Model file for the job. Use its own axes, mm. Face numbers are marked on the shaded views. A direction names the side the tool comes from. Give positions to 0.01 mm unless a question says otherwise; leave off trailing zeros. Order: outer loops, then holes, each group sorted by start corner. A loop starts at its lowest first (then second) coordinate and runs counter-clockwise, first axis right, second up. Notation, with made-up numbers: (42.5, -36) -> (61.5, -36) arc R35 cw to (61.5, 3) -> close; hole circle Ø6 at (-29, 72). An arc over 180 degrees is marked (long way). Use CSV: the item, a comma, the result in double quotes. Start each with the question number.
1. Cut at C-C on y = 3.5. List the corners of the cut face in (x, z).
2. Wall check: line 1 (X direction, y = 7.5, z = -1.6); line 2 (X direction, y = 6, z = -1.6); line 3 (Z direction, x = -1.5, y = 7.5). Give the ranges that are in metal, low to high. Write a range as from..to.
3. 3-axis set-ups, long thin cutter, end or side, ignore diameter. For the marked faces 5, 6 and 7: which of +Z, -Z, +X, -X, +Y, -Y reach the whole face in a straight line?
4. Cut at B-B on y = 7.5. List the corners of the cut face in (x, z), then the cut area to 3 significant figures.
5. Cut at A-A on y = 1.5. List the corners of the cut face in (x, z), then the cut area to 3 significant figures.
6. Pull direction X, two halves, no side cores. Call the marked faces 1, 2, 3 and 4: released by +X, released by -X, zero draft, split by the parting line, or undercut.
7. Drop flat-ended pins along their axis: pin 1 (3 mm diameter, centred on x = 2.5, z = -4, fed in from -Y); pin 2 (1.9 mm diameter, centred on x = 0, y = 1, fed in from +Z); pin 3 (1.2 mm diameter, centred on x = 0, y = 1, fed in from -Z). Give the stop position or say it passes through.
```python
from build123d import *

# Parameters (mm, degrees)
F3_DEPTH = 3
F4_R     = 2


with BuildPart() as f1:
    # F0 (on Right) → F1 (revolve)
    with BuildSketch(Plane.YZ):
        Polygon((0, 0.6), (0, 0), (3, 0), (3, 2.4), (10, 2.4), (10, 8.4), (0, 8.6), (0, 9), (-1, 9), (-1, 7.61980002), (9, 7.41980002), (9, 3.4), (0.4, 3.4), (0.4, 0.6), align=None)
    revolve(axis=Axis((0, 5.8202521418, -1.6), (0, 1, 0)))

    # F2 (on face) → F3 (join, through all)
    with BuildSketch(Plane(origin=(0, 3, 0), x_dir=(-1, 0, 0), z_dir=(0, 1, 0))):
        with BuildLine():
            Line((-1.1618950039, -0.5), (1.1618950039, -0.5))
            ThreePointArc((1.1618950039, -0.5), (0, 0), (-1.1618950039, -0.5))
        make_face()
        with BuildLine():
            ThreePointArc((-1.1618950039, -2.7), (0, -3.2), (1.1618950039, -2.7))
            Line((1.1618950039, -2.7), (-1.1618950039, -2.7))
        make_face()
    extrude(amount=-F3_DEPTH)

    # F4
    f4_edges = [f1.edges().sort_by_distance(p)[0] for p in [
        (0, 9, -10.6198),
        (0, 9, -6.6),
    ]]
    fillet(f4_edges, radius=F4_R)


solid = f1.part
```
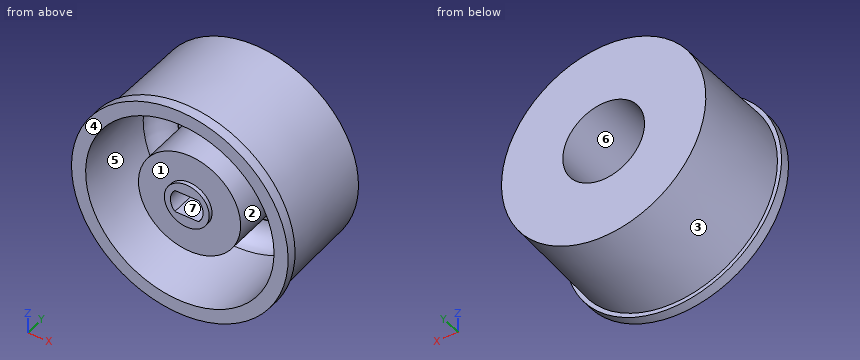
Verdict:
1,outline,"circle Ø20.26 at (0, -1.6); circle Ø10 at (0, -1.6); hole circle Ø18.26 at (0, -1.6); hole circle Ø8 at (0, -1.6)"
2,line 1,"-10.05..-9, -5.06..-4, 4..5.06, 9..10.05"
2,line 2,"-10.08..-9.08, -5..-4, 4..5, 9.08..10.08"
2,line 3,"-11.54..-10.47, -6.44..-5.31, 2.11..3.24, 7.27..8.34"
3,face 5,"-Y"
3,face 6,"+Y"
3,face 7,"+Y, -Y"
4,outline,"circle Ø20.1 at (0, -1.6); circle Ø10.13 at (0, -1.6); hole circle Ø17.99 at (0, -1.6); hole circle Ø8 at (0, -1.6)"
4,area,"93.4 mm^2"
5,outline,"circle Ø20.34 at (0, -1.6); circle Ø10 at (0, -1.6); hole circle Ø18.34 at (0, -1.6); hole (-1.16, -2.7) -> (1.16, -2.7) arc R1.6 ccw to (1.16, -0.5) -> (-1.16, -0.5) arc R1.6 ccw to start"
5,area,"133 mm^2"
6,face 1,"undercut"
6,face 2,"undercut"
6,face 3,"split by the parting line"
6,face 4,"zero draft"
7,pin 1,"y = 0"
7,pin 2,"z = 8.6"
7,pin 3,"z = -11.79"
